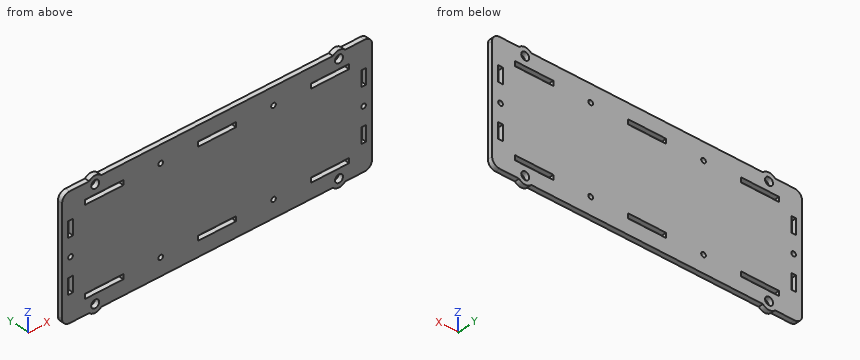
from build123d import *

# Parameters (mm, degrees)
F1_W     = 25.3
F1_H     = 3.2
F1_R     = 1.55
F1_W_2   = 3.2
F1_H_2   = 10.3
F2_DEPTH = 3.2
F4_R     = 5.5
F5_DEPTH = 3.2
F3_R     = 2.65
F6_DEPTH = 3.201
F7_R     = 5


with BuildPart() as f2:
    # F1 (on Front) → F2 (new body)
    with BuildSketch(Plane.XZ):
        Polygon((-99, 81), (-103, 81), (-103, 0), (-99, 0), (99, 0), (103, 0), (103, 81), (99, 81), align=None)
        with Locations((-75, 11.6)):
            Rectangle(F1_W, F1_H, mode=Mode.SUBTRACT)
        with Locations((-37.5, 11.6)):
            Circle(F1_R, mode=Mode.SUBTRACT)
        with Locations((0, 11.6)):
            Rectangle(F1_W, F1_H, mode=Mode.SUBTRACT)
        with Locations((-97.4, 23)):
            Rectangle(F1_W_2, F1_H_2, mode=Mode.SUBTRACT)
        with Locations((37.5, 11.6)):
            Circle(F1_R, mode=Mode.SUBTRACT)
        with Locations((75, 11.6)):
            Rectangle(F1_W, F1_H, mode=Mode.SUBTRACT)
        with Locations((97.4, 23)):
            Rectangle(F1_W_2, F1_H_2, mode=Mode.SUBTRACT)
        with Locations((-97.4, 40.5)):
            Circle(F1_R, mode=Mode.SUBTRACT)
        with Locations((-97.4, 58)):
            Rectangle(F1_W_2, F1_H_2, mode=Mode.SUBTRACT)
        with Locations((-75, 69.4)):
            Rectangle(F1_W, F1_H, mode=Mode.SUBTRACT)
        with Locations((-37.5, 69.4)):
            Circle(F1_R, mode=Mode.SUBTRACT)
        with Locations((0, 69.4)):
            Rectangle(F1_W, F1_H, mode=Mode.SUBTRACT)
        with Locations((97.4, 40.5)):
            Circle(F1_R, mode=Mode.SUBTRACT)
        with Locations((97.4, 58)):
            Rectangle(F1_W_2, F1_H_2, mode=Mode.SUBTRACT)
        with Locations((37.5, 69.4)):
            Circle(F1_R, mode=Mode.SUBTRACT)
        with Locations((75, 69.4)):
            Rectangle(F1_W, F1_H, mode=Mode.SUBTRACT)
    extrude(amount=F2_DEPTH)

    # F4 (on face) → F5 (join, through all)
    with BuildSketch(Plane.XZ.offset(3.2)):
        with Locations((-81, 77.25)):
            Circle(F4_R)
        with Locations((81, 77.25)):
            Circle(F4_R)
        with Locations((81, 3.75)):
            Circle(F4_R)
        with Locations((-81, 3.75)):
            Circle(F4_R)
    extrude(amount=-F5_DEPTH)

    # F3 (on face) → F6 (cut, through all)
    with BuildSketch(Plane.XZ.offset(3.2)):
        with Locations((-81, 77.25)):
            Circle(F3_R)
        with Locations((-81, 3.75)):
            Circle(F3_R)
        with Locations((81, 3.75)):
            Circle(F3_R)
        with Locations((81, 77.25)):
            Circle(F3_R)
    extrude(amount=-F6_DEPTH, mode=Mode.SUBTRACT)

    # F7
    f7_edges = [f2.edges().sort_by_distance(p)[0] for p in [
        (-103, -1.6, 81),
        (-103, -1.6, 0),
        (103, -1.6, 0),
        (103, -1.6, 81),
    ]]
    fillet(f7_edges, radius=F7_R)


solid = f2.part
Geometry check sheet. Reference: the model listing, model coordinates, mm. Give positions to 0.01 mm unless a question says otherwise; leave off trailing zeros. Write each loop counter-clockwise with the first axis right and the second up, starting at its lowest first coordinate (ties: lowest second). Pieces come first, ordered by that corner, then holes. Notation, with made-up numbers: M -33,63.5 L 2,63.5 A19 cw 2,99.5 Z; hole C -39,-21.5 d3. An arc over 180 degrees is marked long. Answer as CSV lines item,"result". Start each with the question number.
Q1. Section check B-B, the plane x = -67.5. Record the cut outline in (y, z).
Q2. Section check A-A, the plane x = 81. Record the cut outline in (y, z).
Q3. Go/stop test with flat-tipped pins: pin 1 (1.5 mm diameter, centred on x = 58, y = -1.5, fed in from +Z); pin 2 (1 mm diameter, centred on x = 97.5, y = -1.5, fed in from -Z). Record where each tip stops, or that it passes through.
Q4. Section check C-C, the plane y = -1.15. Give the number of separate pieces and of enclosed holes in the cut face, then the cut area to 3 significant figures.
Q5. Material ranges on L1, parallel to Z at x = -37.5, y = -1.3; L2, parallel to Z at x = 4.5, y = -2.2; L3, parallel to X at y = -0.45, z = 26, recorded low to high.
Q6. Section check D-D, the plane x = -89.5. Record the cut outline in (y, z), then the cut area to 3 significant figures.
Geometry says:
1,outline,"M -3.2,0 L 0,0 L 0,10 L -3.2,10 Z; M -3.2,13.2 L 0,13.2 L 0,67.8 L -3.2,67.8 Z; M -3.2,71 L 0,71 L 0,81 L -3.2,81 Z"
2,outline,"M -3.2,-1.75 L 0,-1.75 L 0,1.1 L -3.2,1.1 Z; M -3.2,6.4 L 0,6.4 L 0,10 L -3.2,10 Z; M -3.2,13.2 L 0,13.2 L 0,67.8 L -3.2,67.8 Z; M -3.2,71 L 0,71 L 0,74.6 L -3.2,74.6 Z; M -3.2,79.9 L 0,79.9 L 0,82.75 L -3.2,82.75 Z"
3,pin 1,"z = 81"
3,pin 2,"z = 0"
4,separate pieces,"1"
4,enclosed holes,"20"
4,area,"16,000 mm^2"
5,L1,"0 to 10.05, 13.15 to 67.85, 70.95 to 81"
5,L2,"0 to 10, 13.2 to 67.8, 71 to 81"
5,L3,"-103 to -99, -95.8 to 95.8, 99 to 103"
6,outline,"M -3.2,0 L 0,0 L 0,81 L -3.2,81 Z"
6,area,"259 mm^2"
